from build123d import *

# Parameters (mm, degrees)
CYLINDER_R        = 2
CYLINDER_DEPTH    = 14.5
CYLINDER001_R     = 4
CYLINDER001_DEPTH = 14.5


with BuildPart() as cylinder:
    # Cylinder → Cylinder (new body)
    with BuildSketch(Plane.XY):
        Circle(CYLINDER_R)
    extrude(amount=CYLINDER_DEPTH)


with BuildPart() as spacer1:
    # Cylinder001 → Cylinder001 (new body)
    with BuildSketch(Plane.XY):
        Circle(CYLINDER001_R)
    extrude(amount=CYLINDER001_DEPTH)

    # Cut: cut Cylinder
    add(cylinder.part, mode=Mode.SUBTRACT)


with BuildPart() as spacer1_1:
    # Cut placement: moved
    add(spacer1.part.moved(Location((-57, 71, 49))))


solid = spacer1_1.part
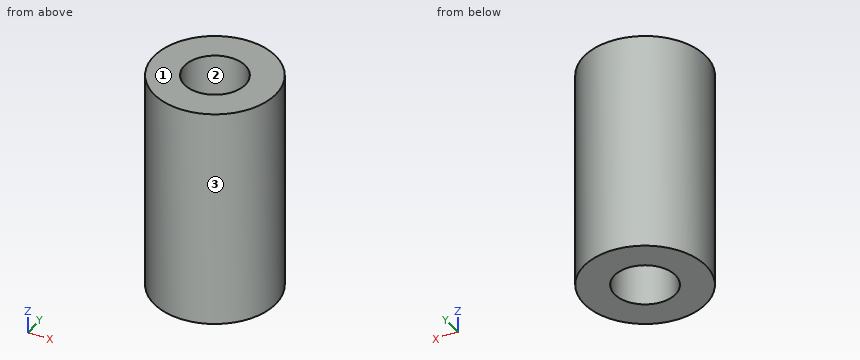
The listing builds one solid part. Answer for the finished solid, in the listing's coordinates (mm). Face numbers are marked on the shaded views. Coordinates: 2 decimals unless noted, no trailing zeros. Write each loop counter-clockwise with the first axis right and the second up, starting at its lowest first coordinate (ties: lowest second). Pieces come first, ordered by that corner, then holes. Notation, with made-up numbers: (84.25, 51) - (109.25, 51) arc R10 ccw to (109.25, 66) - close; hole circle Ø6 at (3.5, -29). An arc over 180 degrees is marked (long way). Return JSON: item names as keys, results as strings.
1. Consider line 1 along Y through (x, z) = (-57, 56); line 2 along X through (y, z) = (71.75, 52.25); line 3 along Y through (x, z) = (-55.75, 57). Determine where each line is inside the solid, lowest interval first.
Final values:
{"line 1": "67 to 69, 73 to 75", "line 2": "-60.93 to -58.85, -55.15 to -53.07", "line 3": "67.2 to 69.44, 72.56 to 74.8"}
2. The part is cut by section B-B on x = -57. Determine the outline of the cut face in (y, z), then the cut area to 3 significant figures.
Final values:
{"outline": "(67, 49) - (69, 49) - (69, 63.5) - (67, 63.5) - close; (73, 49) - (75, 49) - (75, 63.5) - (73, 63.5) - close", "area": "58.0 mm^2"}
3. The part is cut by section A-A on y = 71. Determine the outline of the cut face in (x, z).
Final values:
{"outline": "(-61, 49) - (-59, 49) - (-59, 63.5) - (-61, 63.5) - close; (-55, 49) - (-53, 49) - (-53, 63.5) - (-55, 63.5) - close"}
4. For a pull along Y with two mould halves and no side action, classify the marked faces 1, 2 and 3 as +Y half, -Y half, draft (parallel to the pull), parting line (faces both ways), or undercut.
Final values:
{"face 1": "draft", "face 2": "undercut", "face 3": "parting line"}
5. The part is cut by section C-C on z = 54.75. Determine the outline of the cut face in (x, y).
Final values:
{"outline": "circle Ø8 at (-57, 71); hole circle Ø4 at (-57, 71)"}
6. The part is cut by section D-D on y = 74.25. Determine the outline of the cut face in (x, z).
Final values:
{"outline": "(-59.33, 49) - (-54.67, 49) - (-54.67, 63.5) - (-59.33, 63.5) - close"}
7. Each of these flat-tipped pins is pushed along its axis until it touches: pin 1 Ø2 at (y, z) = (72, 59.5) entering from +X; pin 2 Ø4 at (x, z) = (-54, 55.5) entering from -Y. Where does it stop, or does it pass through?
Final values:
{"pin 1": "x = -53", "pin 2": "y = 67.13"}
